The drawing under review shows one solid part. Ordinate dimensions are in mm from its lowest x, y, z. Coordinates: 2 decimals unless noted, no trailing zeros. Loops run counter-clockwise (first coordinate to the right, second up) from the corner with the lowest first, then second, coordinate; pieces in that order, holes last. Notation, with made-up numbers: M 77,8.25 L 123,8.25 A18 cw 123,14.25 Z; hole C 81,61 d8. An arc over 180 degrees is marked long. Put each result on its own line as item: value.
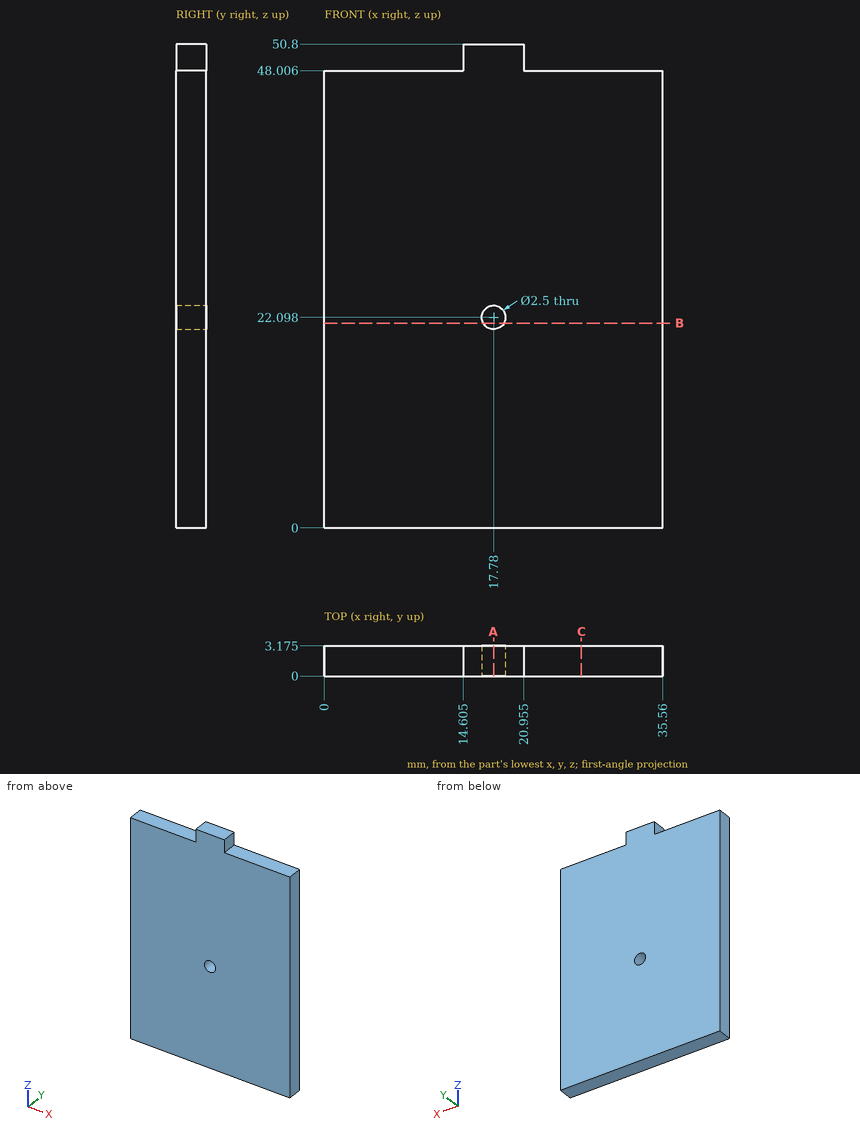
(1) Add section B-B (z = 21.5). Write out the cut boundary in (x, y) (3 decimals).
Determined:
outline: M 0,0 L 16.682,0 L 16.682,3.175 L 0,3.175 Z; M 18.878,0 L 35.56,0 L 35.56,3.175 L 18.878,3.175 Z
(2) Add section C-C (x = 27). Write out the cut boundary in (y, z) (3 decimals), plus the area to 3 significant figures.
Determined:
outline: M 0,0 L 3.175,0 L 3.175,48.006 L 0,48.006 Z
area: 152 mm^2
(3) For pin 1 (1.4 mm diameter, centred on y = 1.5, z = 49.5, fed in from +X) (3 decimals); pin 2 (1.6 mm diameter, centred on x = 26, y = 2.5, fed in from +Z), all flat-tipped, find the tip position at first contact; note any pin that passes through.
Determined:
pin 1: stops at x = 20.955
pin 2: stops at z = 48.01
(4) Wall thickness on line 1 along Z through (x, y) = (17.78, 1.75); line 2 along Z through (x, y) = (22, 0.2); line 3 along X through (y, z) = (1.3, 21): over which ranges is each line inside the solid? List them lowest first. Write a range as [from, to].
Determined:
line 1: z = [0, 20.85], [23.35, 50.8]
line 2: z = [0, 48.01]
line 3: x = [0, 17.18], [18.38, 35.56]
(5) Add section A-A (x = 17.78). Write out the cut boundary in (y, z) (3 decimals), plus the area to 3 significant figures.
Determined:
outline: M 0,0 L 3.175,0 L 3.175,20.848 L 0,20.848 Z; M 0,23.348 L 3.175,23.348 L 3.175,50.8 L 0,50.8 Z
area: 153 mm^2
